The model under review builds one solid part; all positions refer to its coordinate system, in mm. Face numbers are marked on the shaded views. A direction names the side the tool comes from. Give positions to 0.01 mm unless a question says otherwise; leave off trailing zeros. Order: outer loops, then holes, each group sorted by start corner. A loop starts at its lowest first (then second) coordinate and runs counter-clockwise, first axis right, second up. Notation, with made-up numbers: (69, 10.25) - (83, 10.25) arc R28 cw to (83, 28.25) - close; hole circle Ø2 at (-23, 14.25). An arc over 180 degrees is marked (long way). Use a Markdown table: item, result. Add a question column.
```python
from build123d import *

# Parameters (mm, degrees)
SKETCH1_W           = 50.8
SKETCH1_H           = 50.8
BOSS_EXTRUDE1_DEPTH = 177.8
SHELL1_T            = -1.5875
SKETCH2_R           = 2.4892
CUT_EXTRUDE1_DEPTH  = 192.765794656
LPATTERN1_COUNT     = 7
LPATTERN1_PITCH     = 25.4


with BuildPart() as part:
    # Sketch1 → Boss-Extrude1 (new body)
    with BuildSketch(Plane(origin=(0, 0, 0), x_dir=(0, 0, -1), z_dir=(1, 0, 0))):
        with Locations((25.4, 25.4)):
            Rectangle(SKETCH1_W, SKETCH1_H)
    extrude(amount=BOSS_EXTRUDE1_DEPTH)

    # Shell1
    shell1_openings = [part.faces().sort_by_distance(p)[0] for p in [
        (177.8, 25.4, -25.4),
        (0, 25.4, -25.4),
    ]]
    offset(amount=SHELL1_T, openings=shell1_openings, kind=Kind.INTERSECTION)

    # Sketch2 → Cut-Extrude1 (cut, through all)
    with BuildSketch(Plane(origin=(0, 0, -50.8), x_dir=(-1, 0, 0), z_dir=(0, 0, -1))):
        with Locations((-12.7, 12.7)):
            Circle(SKETCH2_R)
        with Locations((-12.7, 38.1)):
            Circle(SKETCH2_R)
    cut_extrude1 = extrude(amount=-CUT_EXTRUDE1_DEPTH, mode=Mode.SUBTRACT)

    # LPattern1: Cut-Extrude1 ×7
    with Locations(*[(i * LPATTERN1_PITCH, 0, 0) for i in range(1, LPATTERN1_COUNT)]):
        add(cut_extrude1, mode=Mode.SUBTRACT)


solid = part.part
```
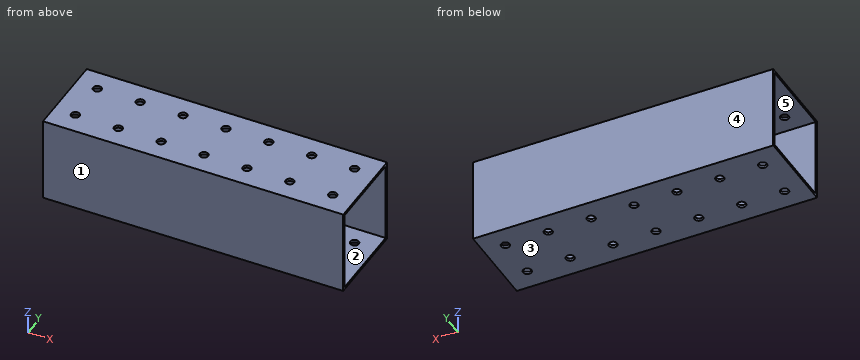
Q1. We need section B-B (z = -27.5). Write out the cut boundary in (x, y), plus the area to 3 significant figures.
Q2. We need section C-C (y = 20.5). Write out the cut boundary in (x, z).
Q3. Wall thickness on probe 1 along Y at (x, z) = (114.3, -50.3); probe 2 along Z at (x, y) = (35.5, 46.5); probe 3 along Y at (x, z) = (158.5, -20): over which ranges is each line inside the solid? List them lowest first.
Q4. Machinability: for the marked faces 4 and 5, which of the approach directions +Z, -Z, +X, -X, +Y, -Y give a long, thin tool a straight path to every point of the face, cutting with its end or side? Answer none if there is none.
Q5. We need section A-A (x = 139.7). Write out the cut boundary in (y, z).
Q6. Draft analysis for pull direction Z (two halves, no side actions). For the marked faces 1, 2 and 3, state which applies: pulls with the +Z half, pulls with the -Z half, needs draft (parallel to the pull), parting line crosses it, or undercut.
Q7. We need section D-D (y = 38.1). Count the separate pieces of the cut face and the enclosed holes in it, plus the area to 3 significant figures.
Here are the results:
| question | item | result |
|---|---|---|
| 1 | outline | (0, 0) - (177.8, 0) - (177.8, 1.59) - (0, 1.59) - close; (0, 49.21) - (177.8, 49.21) - (177.8, 50.8) - (0, 50.8) - close |
| 1 | area | 565 mm2 |
| 2 | outline | (0, -50.8) - (177.8, -50.8) - (177.8, -49.21) - (0, -49.21) - close; (0, -1.59) - (177.8, -1.59) - (177.8, 0) - (0, 0) - close |
| 3 | probe 1 | 0 to 10.21, 15.19 to 35.61, 40.59 to 50.8 |
| 3 | probe 2 | -50.8 to -49.21, -1.59 to 0 |
| 3 | probe 3 | 0 to 1.59, 49.21 to 50.8 |
| 4 | face 4 | +Z, -Z, +X, -X, +Y |
| 4 | face 5 | +X, -X |
| 5 | outline | (0, -50.8) - (10.21, -50.8) - (10.21, -49.21) - (1.59, -49.21) - (1.59, -1.59) - (10.21, -1.59) - (10.21, 0) - (0, 0) - close; (15.19, -50.8) - (35.61, -50.8) - (35.61, -49.21) - (15.19, -49.21) - close; (15.19, -1.59) - (35.61, -1.59) - (35.61, 0) - (15.19, 0) - close; (40.59, -50.8) - (50.8, -50.8) - (50.8, 0) - (40.59, 0) - (40.59, -1.59) - (49.21, -1.59) - (49.21, -49.21) - (40.59, -49.21) - close |
| 6 | face 1 | needs draft |
| 6 | face 2 | undercut |
| 6 | face 3 | pulls with the -Z half |
| 7 | separate pieces | 16 |
| 7 | enclosed holes | 0 |
| 7 | area | 454 mm2 |
